from build123d import *

# Parameters (mm, degrees)
SKETCH2_R               = 4.25
BOSS_EXTRUDE1_DEPTH     = 5.08
CUT_EXTRUDE1_DEPTH      = 32.882966676
CUT_EXTRUDE1_DEPTH_BACK = 32.882966676
SKETCH3_R               = 1.190625


with BuildPart() as part:
    # Sketch1 → Revolve1 (revolve)
    with BuildSketch(Plane.XY, mode=Mode.PRIVATE) as revolve1_sk:
        Polygon((0, 1.5875), (0, 6.35), (-4.87911158, 6.35), (-4.87911158, 20.5), (-8.187387237, 20.5), (-8.187387237, 4.5), (-6.426815736, 4.5), (-6.426815736, 1.5875), align=None)
    revolve(revolve1_sk.sketch.rotate(Axis((0, 0, 0), (-1, 0, 0)), 90), axis=Axis((0, 0, 0), (-1, 0, 0)))

    # Sketch2 → Boss-Extrude1 (add)
    with BuildSketch(Plane.ZY.offset(8.187387237)):
        with Locations(Location((0, 12.6, 0), (0, 0, 180))):
            Circle(SKETCH2_R)
        with Locations(Location((12.6, 0, 0), (0, 0, 180))):
            Circle(SKETCH2_R)
        with Locations(Location((0, -12.6, 0), (0, 0, 180))):
            Circle(SKETCH2_R)
        with Locations(Location((-12.6, 0, 0), (0, 0, 180))):
            Circle(SKETCH2_R)
    extrude(amount=BOSS_EXTRUDE1_DEPTH)

    # Sketch3 → Cut-Extrude1 (cut, two sides: drawn at the far end of the back side and taken through both)
    with BuildSketch(Plane(origin=(0, 0, 0), x_dir=(1, 0, 0), z_dir=(0, 1, 0)).offset(-CUT_EXTRUDE1_DEPTH_BACK)):
        with Locations(Location((-2.623694819, 0, 0), (0, 0, 270))):
            Circle(SKETCH3_R)
    extrude(amount=CUT_EXTRUDE1_DEPTH + CUT_EXTRUDE1_DEPTH_BACK, mode=Mode.SUBTRACT)


solid = part.part
Check sheet for the modelled part. Datum: model origin and axes. Units: mm. A direction names the side the tool comes from. Round coordinates to 2 decimals unless told otherwise and drop trailing zeros. Loops run counter-clockwise (first coordinate to the right, second up) from the corner with the lowest first, then second, coordinate; pieces in that order, holes last.
1. Scan lines: probe 1 along Y at (x, z) = (-7.6, 0); probe 2 along X at (y, z) = (-15, -11); probe 3 along Y at (x, z) = (-4, 0). Record each from-to range of solid material in increasing order.
2. Sectioned sample at A-A on z = 0. Give the number of separate pieces and of enclosed holes in the cut face, and give its area (3 significant figures).
3. Sectioned sample at D-D on z = 12.6. Record the boundary of the cut face in (x, y), and give its area (3 significant figures).
4. Gauge pin test, flat ends, axial feed: pin 1 Ø2.5 at (y, z) = (1.5, 0) entering from -X; pin 2 Ø5 at (x, y) = (-6, -9.5) entering from -Z; pin 3 Ø1 at (y, z) = (5.5, -16.5) entering from +X. Record the tip position at first contact, or that the pin passes through.
5. Mould release check, pull along Z, two halves, no side actions. Record for faces 1 (the cylindrical face through (-2.474, 5.634, -2.93)), 2 (the cylindrical face through (-2.57, -3.74, -1.19)), 3 (the flat face through (-13.267, 0, 13)): released by +Z, released by -Z, zero draft, split by the parting line, or undercut.
6. Set-up check for faces 4 (the cylindrical face through (-7.29, -3.04, 3.32)), 5 (the flat face through (-4.879, -5, -5)), 6 (the flat face through (-13.267, 0, -13)): record each of +Z, -Z, +X, -X, +Y, -Y from which the full face is reachable in a straight line by a thin tool's end or side.
7. Sectioned sample at B-B on y = 0. Record the boundary of the cut face in (x, z), and give its area (3 significant figures).
8. Sectioned sample at C-C on x = -9. Record the boundary of the cut face in (y, z).
Recorded:
1. probe 1: y = -20.5 to -4.5, 4.5 to 20.5
1. probe 2: x = -8.19 to -4.88
1. probe 3: y = -6.35 to -1.59, 1.59 to 6.35
2. separate pieces: 4
2. enclosed holes: 0
2. area: 225 mm2
3. outline: (-13.27, -4.25) - (-8.19, -4.25) - (-8.19, -16.17) - (-4.88, -16.17) - (-4.88, 16.17) - (-8.19, 16.17) - (-8.19, 4.25) - (-13.27, 4.25) - close
3. area: 150 mm2
4. pin 1: stops at x = -6.43
4. pin 2: stops at z = -19.27
4. pin 3: stops at x = -4.88
5. face 1: split by the parting line
5. face 2: undercut
5. face 3: zero draft
6. face 4: -X
6. face 5: +X
6. face 6: +Z, -Z, -X, +Y, -Y
7. outline: (-13.27, -16.85) - (-8.19, -16.85) - (-8.19, -20.5) - (-4.88, -20.5) - (-4.88, -6.35) - (0, -6.35) - (0, -1.59) - (-6.43, -1.59) - (-6.43, -4.5) - (-8.19, -4.5) - (-8.19, -8.35) - (-13.27, -8.35) - close; (-13.27, 8.35) - (-8.19, 8.35) - (-8.19, 4.5) - (-6.43, 4.5) - (-6.43, 1.59) - (0, 1.59) - (0, 6.35) - (-4.88, 6.35) - (-4.88, 20.5) - (-8.19, 20.5) - (-8.19, 16.85) - (-13.27, 16.85) - close
7. area: 248 mm2
8. outline: circle Ø8.5 at (-12.6, 0); circle Ø8.5 at (0, -12.6); circle Ø8.5 at (0, 12.6); circle Ø8.5 at (12.6, 0)
